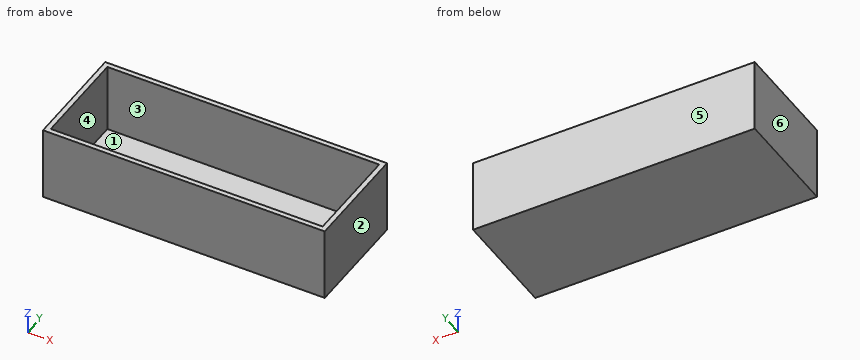
Solid Edge part; units mm, degrees
sketch "Sketch1" plane through (0, 0, 0) normal (0, 0, 1) x (1, 0, 0)
  line L0 (-57.9945, -21.1726) -> (56.0055, -21.1726)
  line L1 (56.0055, -21.1726) -> (56.0055, 22.8274)
  line L2 (56.0055, 22.8274) -> (-57.9945, 22.8274)
  line L3 (-57.9945, 22.8274) -> (-57.9945, -21.1726)
extrude "Protrusion1" add sketch "Sketch1" along normal blind 30
sketch "Sketch2" plane through (-0.9945, 0.8274, 30) normal (0, 0, 1) x (1, 0, 0)
  line L0 (-55, -20) -> (55, -20)
  line L1 (55, -20) -> (55, 20)
  line L2 (55, 20) -> (-55, 20)
  line L3 (-55, 20) -> (-55, -20)
extrude "ExtrudedCutout_1" cut sketch "Sketch2" against normal blind 28
The model under review builds one solid part; all positions refer to its coordinate system, in mm. Face numbers are marked on the shaded views. A direction names the side the tool comes from. Coordinates: 2 decimals unless noted, no trailing zeros. Write each loop counter-clockwise with the first axis right and the second up, starting at its lowest first coordinate (ties: lowest second). Pieces come first, ordered by that corner, then holes. Notation, with made-up numbers: (14.25, 4) - (42.25, 4) arc R13 ccw to (42.25, 10) - close; hole circle Ø5 at (26, 79.5). An arc over 180 degrees is marked (long way). Answer in a Markdown table with one row per item. Add a question column.
Q1. Draft analysis for pull direction Y (two halves, no side actions). For the marked faces 3, 4, 5 and 6, state which applies: +Y half, -Y half, draft (parallel to the pull), parting line (faces both ways), or undercut.
Q2. Consider section A-A on z = 23.75. Give the boundary of the cut face in (x, y).
Q3. For the marked faces 1 and 2, list the 3-axis set-ups (+Z, -Z, +X, -X, +Y, -Y) from which the entire face can be reached by the end or side of a thin tool; tool diameter is ignored.
Q4. Consider section C-C on y = 7. Give the boundary of the cut face in (x, z).
Q5. To check wall thickness, follow line 1 along Y through (x, z) = (51.5, 27); line 2 along X through (y, z) = (-17.5, 15.25); line 3 along Z through (x, y) = (23.5, 15.5). State the ranges of each line that lie inside material, in increasing order. Write a range as from..to.
Q6. Consider section B-B on x = -2.5. Give the boundary of the cut face in (y, z), then the cut area to 3 significant figures.
Q7. Clearance check with flat-ended pins moving along their axes: pin 1 (4 mm diameter, centred on x = 13, y = -6, fed in from +Z); pin 2 (5 mm diameter, centred on x = -33.5, y = 4.5, fed in from -Z). State where each tip first meets the part, or that it passes through.
Answers below:
| question | item | result |
|---|---|---|
| 1 | face 3 | undercut |
| 1 | face 4 | undercut |
| 1 | face 5 | +Y half |
| 1 | face 6 | draft |
| 2 | outline | (-57.99, -21.17) - (56.01, -21.17) - (56.01, 22.83) - (-57.99, 22.83) - close; hole (-55.99, -19.17) - (54.01, -19.17) - (54.01, 20.83) - (-55.99, 20.83) - close |
| 3 | face 1 | +Z |
| 3 | face 2 | +Z, -Z, +X, +Y, -Y |
| 4 | outline | (-57.99, 0) - (56.01, 0) - (56.01, 30) - (54.01, 30) - (54.01, 2) - (-55.99, 2) - (-55.99, 30) - (-57.99, 30) - close |
| 5 | line 1 | -21.17..-19.17, 20.83..22.83 |
| 5 | line 2 | -57.99..-55.99, 54.01..56.01 |
| 5 | line 3 | 0..2 |
| 6 | outline | (-21.17, 0) - (22.83, 0) - (22.83, 30) - (20.83, 30) - (20.83, 2) - (-19.17, 2) - (-19.17, 30) - (-21.17, 30) - close |
| 6 | area | 200 mm² |
| 7 | pin 1 | z = 2 |
| 7 | pin 2 | z = 0 |
